```python
from build123d import *
from OCP.BRepFilletAPI import BRepFilletAPI_MakeChamfer

# Parameters (mm, degrees)
SKETCH1_W           = 50.8
SKETCH1_H           = 50.8
BOSS_EXTRUDE1_DEPTH = 50.8
CUT_EXTRUDE1_DEPTH  = 50.8
SKETCH4_R           = 3.175
CUT_EXTRUDE2_DEPTH  = 12.7
SKETCH5_R           = 3.175
CUT_EXTRUDE3_DEPTH  = 12.7
CHAMFER1_SIZE       = 0.508
CHAMFER3_SIZE       = 0.508
CHAMFER3_SIZE2      = 1.38788181
FILLET3_R           = 7.62
BOSS_EXTRUDE2_DEPTH = 50.8
CHAMFER4_SIZE       = 0.508
CHAMFER5_SIZE       = 0.508
SKETCH7_R           = 3.079866406
SKETCH7_R_2         = 3.504854353
CUT_EXTRUDE4_DEPTH  = 19.05
SKETCH9_W           = 60.012063762
SKETCH9_H           = 6.35
BOSS_EXTRUDE4_DEPTH = 12.7
SKETCH10_W          = 6.35
SKETCH10_H          = 37.305371191
BOSS_EXTRUDE5_DEPTH = 12.7
FILLET6_R           = 5.08


with BuildPart() as part:
    # Sketch1 → Boss-Extrude1 (new body)
    with BuildSketch(Plane.XY):
        Rectangle(SKETCH1_W, SKETCH1_H)
    extrude(amount=BOSS_EXTRUDE1_DEPTH)

    # Sketch2 → Cut-Extrude1 (cut)
    with BuildSketch(Plane.XY.offset(50.8)):
        Polygon((-25.4, 18.594090512), (0, -25.4), (-25.4, -25.4), align=None)
    extrude(amount=-CUT_EXTRUDE1_DEPTH, mode=Mode.SUBTRACT)

    # Sketch4 → Cut-Extrude2 (cut)
    with BuildSketch(Plane(origin=(25.4, 0, 0), x_dir=(0, 0, -1), z_dir=(1, 0, 0))):
        with Locations((-44.45, 19.05)):
            Circle(SKETCH4_R)
        with Locations((-6.35, 19.05)):
            Circle(SKETCH4_R)
        with Locations((-6.35, -19.05)):
            Circle(SKETCH4_R)
        with Locations((-44.45, -19.05)):
            Circle(SKETCH4_R)
    extrude(amount=-CUT_EXTRUDE2_DEPTH, mode=Mode.SUBTRACT)

    # Sketch5 → Cut-Extrude3 (cut)
    with BuildSketch(Plane(origin=(-10.998522628, -6.35, 0), x_dir=(0, 0, 1), z_dir=(-0.8660254037844364, -0.5000000000000041, 0))):
        with Locations(Location((6.35, 22.452954744, 0), (0, 0, 270))):
            Circle(SKETCH5_R)
        with Locations(Location((44.45, 22.452954744, 0), (0, 0, 270))):
            Circle(SKETCH5_R)
        with Locations(Location((44.45, -15.647045256, 0), (0, 0, 270))):
            Circle(SKETCH5_R)
        with Locations(Location((6.35, -15.647045256, 0), (0, 0, 270))):
            Circle(SKETCH5_R)
    extrude(amount=-CUT_EXTRUDE3_DEPTH, mode=Mode.SUBTRACT)

    # Chamfer1
    chamfer1_edges = [part.edges().sort_by_distance(p)[0] for p in [
        (25.4, -19.05, 47.625),
        (25.4, -19.05, 9.525),
        (25.4, 19.05, 9.525),
        (25.4, 19.05, 47.625),
        (25.4, 0, 50.8),
        (25.4, 0, 0),
        (25.4, -25.4, 25.4),
        (25.4, 25.4, 25.4),
    ]]
    chamfer(chamfer1_edges, length=CHAMFER1_SIZE)

    # Chamfer3: one chamfer whose edges measure the first distance from different faces: ONE call of the kernel's chamfer builder (chamfer() names one face for all edges)
    chamfer3_edges_1 = [part.edges().sort_by_distance(p)[0] for p in [
        (0, -25.4, 25.4),
    ]]
    chamfer3_side_1 = [part.faces().sort_by_distance(p)[0] for p in [
        (12.446, -25.4, 25.4),
    ]]
    chamfer3_edges_2 = [part.edges().sort_by_distance(p)[0] for p in [
        (-4.7625, -17.151108029, 6.35),
        (-4.7625, -17.151108029, 44.45),
        (-23.8125, 15.844459855, 44.45),
        (-23.8125, 15.844459855, 6.35),
    ]]
    chamfer3 = BRepFilletAPI_MakeChamfer(part.part.solid().wrapped)
    for e in chamfer3_edges_1:
        chamfer3.Add(CHAMFER3_SIZE, CHAMFER3_SIZE2, e.wrapped, chamfer3_side_1[0].wrapped)  # the first distance lies on this face
    for e in chamfer3_edges_2:
        chamfer3.Add(CHAMFER3_SIZE, e.wrapped)
    add(Compound.cast(chamfer3.Shape()), mode=Mode.REPLACE)

    # Fillet3
    fillet3_edges = [part.edges().sort_by_distance(p)[0] for p in [
        (-25.4, 18.594090512, 25.4),
    ]]
    fillet(fillet3_edges, radius=FILLET3_R)

    # Sketch6 → Boss-Extrude2 (add, through all)
    with BuildSketch(Plane(origin=(0, 0, 0), x_dir=(-1, 0, 0), z_dir=(0, 0, -1))):
        Polygon((18.145405324, 59.69), (-12.192, 25.4), (-3.713506547, 25.4), (21.005860753, 53.34), (119.117924515, 53.34), (119.117924515, 59.69), align=None)
    extrude(amount=-BOSS_EXTRUDE2_DEPTH)

    # Chamfer4
    # the kernel refuses this chamfer: 0.508 mm, written as the material it takes off along each edge
    with BuildSketch(Plane(origin=(-0.798414958, -25.4, 0), x_dir=(0, 0.9996219169112968, -0.027495876610586417), z_dir=(1, 0, 0)), Plane(origin=(-0.798414958, -25.4, 50.8), x_dir=(0, -0.027495876610587118, -0.9996219169112968), z_dir=(1, 0, 0))) as chamfer4_piece_1:
        Polygon((CHAMFER4_SIZE * 0.999621916911, CHAMFER4_SIZE * 0.0274958766106), (-CHAMFER4_SIZE * 0.0274958766106, CHAMFER4_SIZE * 0.999621916911), (0, 0), align=None)
    extrude(amount=26.996829916, mode=Mode.SUBTRACT)
    with BuildSketch(Plane(origin=(-25.4, 26.706414958, 50.8), x_dir=(-0.027495876610587118, 0, -0.9996219169112968), z_dir=(0, -1, 0)), Plane(origin=(-25.4, 26.706414958, 0), x_dir=(0.9996219169112968, 0, -0.027495876610586417), z_dir=(0, -1, 0))) as chamfer4_piece_2:
        Polygon((CHAMFER4_SIZE * 0.999621916911, CHAMFER4_SIZE * 0.0274958766106), (-CHAMFER4_SIZE * 0.0274958766106, CHAMFER4_SIZE * 0.999621916911), (0, 0), align=None)
    extrude(amount=6.070551599, mode=Mode.SUBTRACT)
    with BuildSketch(Plane(origin=(-17.78, 20.635863359, 50.8), x_dir=(-0.8660254037844363, -0.5000000000000041, 0), z_dir=(0.5000000000000041, -0.8660254037844363, 0))) as chamfer4_piece_3:
        Polygon((7.62, CHAMFER4_SIZE), (7.62 - CHAMFER4_SIZE, 0), (7.62, 0), align=None)
    revolve(axis=Axis((-17.78, 20.635863359, 50.8), (0, 0, -1)), revolution_arc=30, mode=Mode.SUBTRACT)
    with BuildSketch(Plane(origin=(-24.379113577, 16.825863359, 50.8), x_dir=(-0.023812127644096983, -0.013747938305297273, -0.9996219169112965), z_dir=(0.5000000000000041, -0.8660254037844363, 0)), Plane(origin=(-24.379113577, 16.825863359, 0), x_dir=(0.8656979742248779, 0.4998109584556525, -0.027495876610586285), z_dir=(0.5000000000000041, -0.8660254037844363, 0))) as chamfer4_piece_4:
        Polygon((CHAMFER4_SIZE * 0.999621916911, CHAMFER4_SIZE * 0.0274958766106), (-CHAMFER4_SIZE * 0.0274958766106, CHAMFER4_SIZE * 0.999621916911), (0, 0), align=None)
    extrude(amount=48.676760301, mode=Mode.SUBTRACT)
    with BuildSketch(Plane(origin=(-17.78, 20.635863359, 0), x_dir=(-0.8660254037844363, -0.5000000000000041, 0), z_dir=(0.5000000000000041, -0.8660254037844363, 0))) as chamfer4_piece_5:
        Polygon((7.62 - CHAMFER4_SIZE, 0), (7.62, -CHAMFER4_SIZE), (7.62, 0), align=None)
    revolve(axis=Axis((-17.78, 20.635863359, 0), (0, 0, -1)), revolution_arc=30, mode=Mode.SUBTRACT)

    # Chamfer5
    chamfer5_edges = [part.edges().sort_by_distance(p)[0] for p in [
        (-8.646177103, 39.37, 0),
        (-2.976702662, 42.545, 0),
        (-8.646177103, 39.37, 50.8),
        (-2.976702662, 42.545, 50.8),
    ]]
    chamfer(chamfer5_edges, length=CHAMFER5_SIZE)

    # Sketch7 → Cut-Extrude4 (cut)
    with BuildSketch(Plane(origin=(0, 59.69, 0), x_dir=(1, 0, 0), z_dir=(0, 1, 0))):
        with Locations(Location((-100.067924515, -6.35, 0), (0, 0, 270))):
            Circle(SKETCH7_R)
        with Locations(Location((-100.067924515, -44.45, 0), (0, 0, 270))):
            Circle(SKETCH7_R_2)
    extrude(amount=-CUT_EXTRUDE4_DEPTH, mode=Mode.SUBTRACT)

    # Sketch9 → Boss-Extrude4 (add)
    with BuildSketch(Plane(origin=(0, 53.34, 0), x_dir=(-1, 0, 0), z_dir=(0, -1, 0))):
        with Locations((51.011892634, -25.4)):
            Rectangle(SKETCH9_W, SKETCH9_H)
    extrude(amount=BOSS_EXTRUDE4_DEPTH)

    # Sketch10 → Boss-Extrude5 (add)
    with BuildSketch(Plane(origin=(14.688369002, 12.995246543, 0), x_dir=(0, 0, 1), z_dir=(-0.7489538130165907, -0.6626222045539297, 0))):
        with Locations((25.4, 35.215460552)):
            Rectangle(SKETCH10_W, SKETCH10_H)
    extrude(amount=BOSS_EXTRUDE5_DEPTH)

    # Fillet6
    fillet6_edges = [part.edges().sort_by_distance(p)[0] for p in [
        (-51.011892634, 53.34, 22.225),
        (-8.646177103, 39.37, 22.225),
        (-8.646177103, 39.37, 28.575),
        (-51.011892634, 53.34, 28.575),
        (-13.243480358, 25.4, 25.4),
        (3.713506547, 25.4, 39.4335),
        (3.713506547, 25.4, 11.3665),
        (-21.005860753, 53.34, 39.4335),
        (-21.005860753, 53.34, 11.3665),
        (-18.145405324, 59.69, 25.4),
        (12.192, 25.4, 25.4),
    ]]
    fillet(fillet6_edges, radius=FILLET6_R)


solid = part.part
```
Design review of the part built by this model. Coordinates are the model's own, in mm. A direction names the side the tool comes from. Coordinates: 2 decimals unless noted, no trailing zeros. Order: outer loops, then holes, each group sorted by start corner. A loop starts at its lowest first (then second) coordinate and runs counter-clockwise, first axis right, second up.
1) Take a section at A-A, the plane z = 24. Give the boundary of the cut face in (x, y), and give its area (3 significant figures).
2) Take a section at C-C, the plane y = 1.5. Give the boundary of the cut face in (x, z).
3) For faces 1 (the cylindrical face through (-2.966, 28.319, 39.586)), 2 (the flat face through (-2.69, 41.88, 50.52)), 3 (the flat face through (7.8, -13.51, 6.39)), 4 (the cylindrical face through (-2.9, 28.47, 11.52)), 5 (the cylindrical face through (18.88, 17.83, 41.52)), list the 3-axis set-ups (+Z, -Z, +X, -X, +Y, -Y) from which the entire face can be reached by the end or side of a thin tool; tool diameter is ignored.
4) Take a section at B-B, the plane x = -62.5. Give the boundary of the cut face in (y, z) (3 decimals), and give its area (3 significant figures).
5) Take a section at D-D, the plane z = 36. Give the boundary of the cut face in (x, y).
6) Wall thickness on line 1 along Z through (x, y) = (18, 19); line 2 along Y through (x, z) = (19, 6.35) (3 decimals); line 3 along Y through (x, z) = (-82.5, 17.5): over which ranges is each line inside the solid? List them lowest first.
7) Mouldability with a two-part tool opening along X and no side actions: class faces 6 (the cylindrical face through (-21.18, 52.88, 8.94)), 7 (the cylindrical face through (18.88, 15.95, 7.04)), 8 (the cylindrical face through (-16.8, 16.7, 9.5)), 9 (the flat face through (25.4, 0, 25)) as +X half, -X half, draft (parallel to the pull), parting line (faces both ways), or undercut.
8) Clearance check with flat-ended pins moving along their axes: pin 1 (8.5 mm diameter, centred on y = 19.05, z = 6.35, fed in from -X); pin 2 (18.5 mm diameter, centred on x = -59.5, y = 33.5, fed in from +Z) (3 decimals); pin 3 (14.5 mm diameter, centred on x = 16.5, z = 22, fed in from +Y). State where each tip first meets the part, or that it passes through.
Returned:
1. outline: (-119.12, 53.34) - (-81.02, 53.34) - (-81.02, 40.64) - (-26.73, 40.64) - (-20.72, 33.85) arc R5.08 cw to (-24.52, 25.4) - (-25.4, 25.4) - (-25.4, 20.64) arc R7.62 ccw to (-24.38, 16.83) - (-0.69, -24.2) - (0.51, -25.4) - (24.89, -25.4) - (25.4, -24.89) - (25.4, 24.89) - (24.89, 25.4) - (14.48, 25.4) arc R5.08 cw to (10.68, 27.11) - (-16.63, 57.98) arc R5.08 ccw to (-20.43, 59.69) - (-119.12, 59.69) - close
1. area: 4,040 mm2
2. outline: (-15.53, 0.51) - (-14.94, 0) - (24.89, 0) - (25.4, 0.51) - (25.4, 50.29) - (24.89, 50.8) - (-14.94, 50.8) - (-15.53, 50.29) - close
3. face 1: +Z, -X
3. face 2: +Z, +X, +Y
3. face 3: none
3. face 4: -Z, -X
3. face 5: +X
4. outline: (40.64, 22.225) - (48.26, 22.225) arc R5.08 cw to (53.34, 17.145) - (53.34, 0) - (59.69, 0) - (59.69, 50.8) - (53.34, 50.8) - (53.34, 33.655) arc R5.08 cw to (48.26, 28.575) - (40.64, 28.575) - close
4. area: 414 mm2
5. outline: (-119.12, 53.34) - (-23.29, 53.34) arc R5.08 cw to (-19.49, 51.63) - (-3.76, 33.85) arc R5.08 cw to (-7.56, 25.4) - (-25.4, 25.4) - (-25.4, 20.64) arc R7.62 ccw to (-24.38, 16.83) - (-0.69, -24.2) - (0.51, -25.4) - (24.89, -25.4) - (25.4, -24.89) - (25.4, 24.89) - (24.89, 25.4) - (14.48, 25.4) arc R5.08 cw to (10.68, 27.11) - (-16.63, 57.98) arc R5.08 ccw to (-20.43, 59.69) - (-119.12, 59.69) - close
6. line 1: z = 0 to 3.18, 9.52 to 41.28, 47.62 to 50.8
6. line 2: y = -25.4 to -22.225, -15.875 to 15.875, 22.225 to 25.4
6. line 3: y = 53.34 to 59.69
7. face 6: -X half
7. face 7: draft
7. face 8: undercut
7. face 9: +X half
8. pin 1: stops at x = -25.4
8. pin 2: stops at z = 28.575
8. pin 3: stops at y = 28.73
